from build123d import *

# Parameters (mm, degrees)
SKETCH1_W           = 361.95
SKETCH1_H           = 50.8
SKETCH1_R           = 2.286
SKETCH1_R_2         = 10.795
BOSS_EXTRUDE1_DEPTH = 3.175
CUT_EXTRUDE1_DEPTH  = 366.511317369
FILLET1_R           = 12.7
CUT_EXTRUDE2_DEPTH  = 366.511317369
SKETCH4_R           = 2.286
CUT_EXTRUDE3_DEPTH  = 366.511317369
SKETCH6_R           = 2.286
CUT_EXTRUDE4_DEPTH  = 366.511317369


with BuildPart() as part:
    # Sketch1 → Boss-Extrude1 (new body)
    with BuildSketch(Plane.XY):
        with Locations((-180.975, 25.4)):
            Rectangle(SKETCH1_W, SKETCH1_H)
        with Locations((-41.91, 6.35)):
            Circle(SKETCH1_R, mode=Mode.SUBTRACT)
        with Locations((-292.735, 6.35)):
            Circle(SKETCH1_R, mode=Mode.SUBTRACT)
        with Locations((-128.905, 19.05)):
            Circle(SKETCH1_R, mode=Mode.SUBTRACT)
        with Locations((-205.74, 19.05)):
            Circle(SKETCH1_R, mode=Mode.SUBTRACT)
        with Locations((-167.3225, 34.29)):
            Circle(SKETCH1_R_2, mode=Mode.SUBTRACT)
        with Locations((-250.085181934, 18.50662125)):
            Circle(SKETCH1_R, mode=Mode.SUBTRACT)
        with Locations(Location((-84.559818066, 18.50662125, 0), (0, 0, 180))):
            Circle(SKETCH1_R, mode=Mode.SUBTRACT)
    extrude(amount=BOSS_EXTRUDE1_DEPTH)

    # Sketch2 → Cut-Extrude1 (cut, through all)
    with BuildSketch(Plane.XY.offset(3.175)):
        Polygon((-388.62, 50.8), (-337.82, 0), (-388.62, 0), align=None)
    extrude(amount=-CUT_EXTRUDE1_DEPTH, mode=Mode.SUBTRACT)

    # Fillet1
    fillet1_edges = [part.edges().sort_by_distance(p)[0] for p in [
        (-337.82, 0, 1.5875),
        (-361.95, 24.13, 1.5875),
    ]]
    fillet(fillet1_edges, radius=FILLET1_R)

    # Sketch3 → Cut-Extrude2 (cut, through all)
    with BuildSketch(Plane.XY.offset(3.175)):
        Polygon((-256.54, 0), (-205.74, 6.35), (-128.905, 6.35), (-78.105, 0), align=None)
    extrude(amount=-CUT_EXTRUDE2_DEPTH, mode=Mode.SUBTRACT)

    # Sketch4 → Cut-Extrude3 (cut, through all)
    with BuildSketch(Plane(origin=(0, 0, 0), x_dir=(-1, 0, 0), z_dir=(0, 0, -1))):
        with Locations((110.1725, 46.99)):
            Circle(SKETCH4_R)
        with Locations((167.3225, 11.43)):
            Circle(SKETCH4_R)
        with Locations((224.4725, 46.99)):
            Circle(SKETCH4_R)
    extrude(amount=-CUT_EXTRUDE3_DEPTH, mode=Mode.SUBTRACT)

    # Sketch6 → Cut-Extrude4 (cut, through all)
    with BuildSketch(Plane.XY.offset(3.175)):
        with Locations((-72.39, 46.99)):
            Circle(SKETCH6_R)
        with Locations((-10.16, 46.99)):
            Circle(SKETCH6_R)
    extrude(amount=-CUT_EXTRUDE4_DEPTH, mode=Mode.SUBTRACT)


solid = part.part
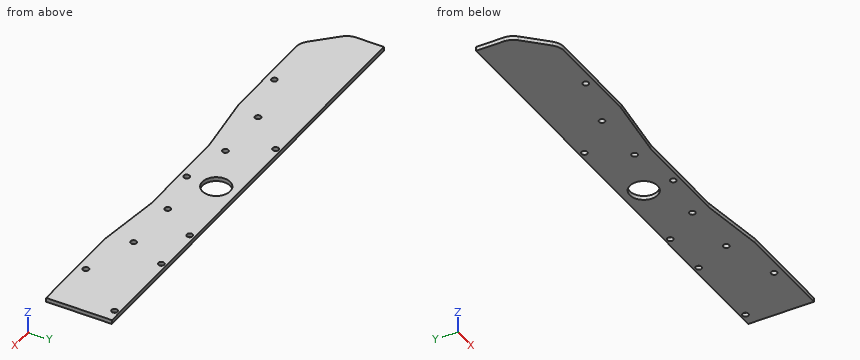
Model file for the job. Use its own axes, mm. Give positions to 0.01 mm unless a question says otherwise; leave off trailing zeros. Order: outer loops, then holes, each group sorted by start corner. A loop starts at its lowest first (then second) coordinate and runs counter-clockwise, first axis right, second up. Notation, with made-up numbers: (67.5, 50) - (114.5, 50) arc R7 cw to (114.5, 60) - close; hole circle Ø9 at (3.5, -34.75). An arc over 180 degrees is marked (long way). Write item = value, one per line. Start each with the question number.
1. Cut at C-C, the plane x = -103.5. List the corners of the cut face in (y, z) (3 decimals).
2. Drop a flat-ended pin along its axis: P1, Ø1.6, axis at x = -158, z = 2, coming from the -Y side. Give the stop position or say it passes through.
3. Cut at A-A, the plane z = 1.4. State how many separate pieces and enclosed holes the cut face has, and give its area (3 significant figures).
4. Cut at B-B, the plane x = -337. List the corners of the cut face in (y, z) (3 decimals).
5. Probe line 1 along X through (y, z) = (48, 1.2); line 2 along X through (y, z) = (46, 2.15); line 3 along X through (y, z) = (11.5, 0.45). List the from-to ranges inside material, lowest first.
Taken from the geometry:
q1.outline = (3.174, 0) - (50.8, 0) - (50.8, 3.175) - (3.174, 3.175) - close
q2.P1 = 6.35
q3.separate_pieces = 1
q3.enclosed_holes = 12
q3.area = 16,700 mm²
q4.outline = (0.802, 0) - (50.8, 0) - (50.8, 3.175) - (0.802, 3.175) - close
q5.line_1 = -361.95 to -226.52, -222.42 to -112.22, -108.12 to -74.44, -70.34 to -12.21, -8.11 to 0
q5.line_2 = -361.95 to -226.53, -222.41 to -112.23, -108.11 to -74.45, -70.33 to -12.22, -8.1 to 0
q5.line_3 = -349.32 to -169.61, -165.04 to 0
